```python
from build123d import *

# Parameters (mm, degrees)
SKETCH_1_W                = 40
SKETCH_1_H                = 70
EXTRUDE_1_DEPTH           = 6
CUT_EXTRUDE_1_DEPTH       = 54.488316481
HOLE_WIZARD_2_D           = 3.4
HOLE_WIZARD_2_CBORE_D     = 6
HOLE_WIZARD_2_CBORE_DEPTH = 3.4


with BuildPart() as part:
    # 草图1 → 凸台-拉伸1 (new body)
    with BuildSketch(Plane(origin=(0, 0, 0), x_dir=(1, 0, 0), z_dir=(0, 1, 0))):
        Rectangle(SKETCH_1_W, SKETCH_1_H)
    extrude(amount=EXTRUDE_1_DEPTH)

    # 草图4 → 切除-拉伸1 (cut, through all)
    with BuildSketch(Plane(origin=(20, 0, 0), x_dir=(0, 0, -1), z_dir=(1, 0, 0))):
        Polygon((-34, 6), (-33.422649731, 5), (-32.845299462, 6), align=None)
        Polygon((-32, 6), (-30.845299462, 6), (-31.422649731, 5), align=None)
        Polygon((-30, 6), (-28.845299462, 6), (-29.422649731, 5), align=None)
        Polygon((-28, 6), (-26.845299462, 6), (-27.422649731, 5), align=None)
        Polygon((-26, 6), (-24.845299462, 6), (-25.422649731, 5), align=None)
        Polygon((-24, 6), (-22.845299462, 6), (-23.422649731, 5), align=None)
        Polygon((-22, 6), (-20.845299462, 6), (-21.422649731, 5), align=None)
        Polygon((-20, 6), (-18.845299462, 6), (-19.422649731, 5), align=None)
        Polygon((-18, 6), (-16.845299462, 6), (-17.422649731, 5), align=None)
        Polygon((-16, 6), (-14.845299462, 6), (-15.422649731, 5), align=None)
        Polygon((-14, 6), (-12.845299462, 6), (-13.422649731, 5), align=None)
        Polygon((-12, 6), (-10.845299462, 6), (-11.422649731, 5), align=None)
        Polygon((-10, 6), (-8.845299462, 6), (-9.422649731, 5), align=None)
        Polygon((-8, 6), (-6.845299462, 6), (-7.422649731, 5), align=None)
        Polygon((-6, 6), (-4.845299462, 6), (-5.422649731, 5), align=None)
        Polygon((-4, 6), (-2.845299462, 6), (-3.422649731, 5), align=None)
        Polygon((-2, 6), (-0.845299462, 6), (-1.422649731, 5), align=None)
        Polygon((0, 6), (1.154700538, 6), (0.577350269, 5), align=None)
        Polygon((2, 6), (3.154700538, 6), (2.577350269, 5), align=None)
        Polygon((4, 6), (5.154700538, 6), (4.577350269, 5), align=None)
    extrude(amount=-CUT_EXTRUDE_1_DEPTH, mode=Mode.SUBTRACT)

    # 打孔尺寸(%根据)内六角圆柱头螺钉的类型2 (through all)
    with Locations(Plane(origin=(-12, 0, -30), x_dir=(0, 0, -1), z_dir=(0, -1, 0))):
        with Locations((0, 0), (0, 12), (0, 24)):
            CounterBoreHole(HOLE_WIZARD_2_D / 2, HOLE_WIZARD_2_CBORE_D / 2, HOLE_WIZARD_2_CBORE_DEPTH)


solid = part.part
```
Geometry check sheet. Reference: the model listing, model coordinates, mm. A direction names the side the tool comes from. Round coordinates to 2 decimals unless told otherwise and drop trailing zeros. Order: outer loops, then holes, each group sorted by start corner. A loop starts at its lowest first (then second) coordinate and runs counter-clockwise, first axis right, second up. Notation, with made-up numbers: (-38, 56.5) -> (3, 56.5) arc R19 cw to (3, 77.5) -> close; hole circle Ø11 at (14, 18.25). An arc over 180 degrees is marked (long way). Return JSON: item names as keys, results as strings. Group by question number.
Q1. Material ranges on probe 1 along X at (y, z) = (4.1, -30); probe 2 along X at (y, z) = (0.9, -30); probe 3 along Z at (x, y) = (11.5, 4), recorded low to high. Write a range as from..to.
Q2. Release check for a two-part mould opening along Z. For faces 3 (the cylindrical face through (-12.65, 4.72, -28.43)), 4 (the flat face through (0, 3, 35)), 5 (the flat face through (-20, 3, 0)) record: released by +Z, released by -Z, zero draft, split by the parting line, or undercut.
Q3. Gauge pin test, flat ends, axial feed: pin 1 (10 mm diameter, centred on x = -12, z = -17, fed in from -Y); pin 2 (5.5 mm diameter, centred on x = 0, z = -30, fed in from -Y); pin 3 (3 mm diameter, centred on x = 12, z = -30, fed in from +Y). Record the tip position at first contact, or that the pin passes through.
Q4. Tool access check on faces 1 (the flat face through (0, 3, -35)), 2 (the cylindrical face through (12, 2, -27)). Record the directions out of +Z, -Z, +X, -X, +Y, -Y that give a thin tool (end or side, any length) a straight path to the whole face; none if there is none.
Q5. Section check A-A, the plane z = -30. Record the boundary of the cut face in (x, y), plus the area to 3 significant figures.
Numbers:
{
 "1": {"probe 1": "-20..-13.7, -10.3..-1.7, 1.7..10.3, 13.7..20", "probe 2": "-20..-15, -9..-3, 3..9, 15..20", "probe 3": "-35..-31.62, -28.38..35"},
 "2": {"face 3": "undercut", "face 4": "released by +Z", "face 5": "zero draft"},
 "3": {"pin 1": "y = 0", "pin 2": "y = 3.4", "pin 3": "through"},
 "4": {"face 1": "-Z, +X, -X, +Y, -Y", "face 2": "-Y"},
 "5": {"outline": "(-20, 0) -> (-15, 0) -> (-15, 3.4) -> (-13.7, 3.4) -> (-13.7, 6) -> (-20, 6) -> close; (-10.3, 3.4) -> (-9, 3.4) -> (-9, 0) -> (-3, 0) -> (-3, 3.4) -> (-1.7, 3.4) -> (-1.7, 6) -> (-10.3, 6) -> close; (1.7, 3.4) -> (3, 3.4) -> (3, 0) -> (9, 0) -> (9, 3.4) -> (10.3, 3.4) -> (10.3, 6) -> (1.7, 6) -> close; (13.7, 3.4) -> (15, 3.4) -> (15, 0) -> (20, 0) -> (20, 6) -> (13.7, 6) -> close", "area": "152 mm^2"}
}
